Design review of the part shown in the three views and the two pictorial views. Dimensions are in mm from the part's minimum x, y and z. Coordinates: 2 decimals unless noted, no trailing zeros. Write each loop counter-clockwise with the first axis right and the second up, starting at its lowest first coordinate (ties: lowest second). Pieces come first, ordered by that corner, then holes. Notation, with made-up numbers: (52.25, 72) -> (80.25, 72) arc R10 ccw to (80.25, 87) -> close; hole circle Ø2 at (11, 64.25). An arc over 180 degrees is marked (long way). Answer in a Markdown table with one row per item. Add a question column.
Item 1: Take a section at A-A, the plane x = 5. Write out the cut boundary in (y, z).
Item 2: Clearance check with a flat-ended pin moving along its axis: P1, Ø6, axis at x = 5, z = 5, coming from the +Y side. State where the tip first meets the part, or that it passes through.
Item 3: To check wall thickness, follow line 1 (X direction, y = 1.15, z = 1); line 2 (Y direction, x = 10.25, z = 14); line 3 (Z direction, x = 6.25, y = 1.7). State the ranges of each line that lie inside material, in increasing order.
Item 4: Take a section at C-C, the plane y = 1.25. Write out the cut boundary in (x, z), and give its area (4 significant figures).
Item 5: Take a section at B-B, the plane z = 6. Write out the cut boundary in (x, y), and give its area (4 significant figures).
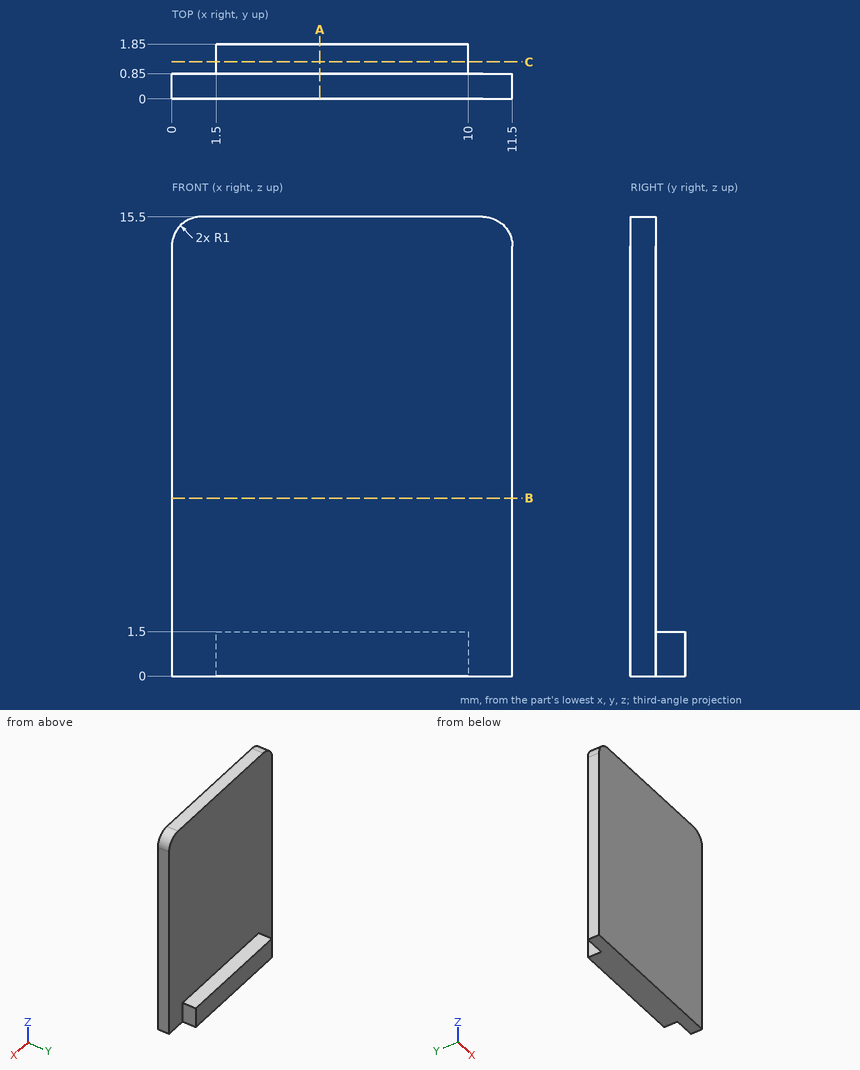
Answers:
| question | item | result |
|---|---|---|
| 1 | outline | (0, 0) -> (1.85, 0) -> (1.85, 1.5) -> (0.85, 1.5) -> (0.85, 15.5) -> (0, 15.5) -> close |
| 2 | P1 | stops at y = 0.85 |
| 3 | line 1 | x = 1.5 to 10 |
| 3 | line 2 | y = 0 to 0.85 |
| 3 | line 3 | z = 0 to 1.5 |
| 4 | outline | (1.5, 0) -> (10, 0) -> (10, 1.5) -> (1.5, 1.5) -> close |
| 4 | area | 12.75 mm^2 |
| 5 | outline | (0, 0) -> (11.5, 0) -> (11.5, 0.85) -> (0, 0.85) -> close |
| 5 | area | 9.775 mm^2 |
